The figure shows three views and two pictorial views of one solid part (mm, origin at its lowest corner). Answer the questions. A direction names the side the tool comes from. Coordinates: 2 decimals unless noted, no trailing zeros. Order: outer loops, then holes, each group sorted by start corner. A loop starts at its lowest first (then second) coordinate and runs counter-clockwise, first axis right, second up. Notation, with made-up numbers: (40, -36) -> (88, -36) arc R23 ccw to (88, -10) -> close; hole circle Ø10 at (-12.75, 8). An arc over 180 degrees is marked (long way). Return JSON: item names as keys, results as strings.
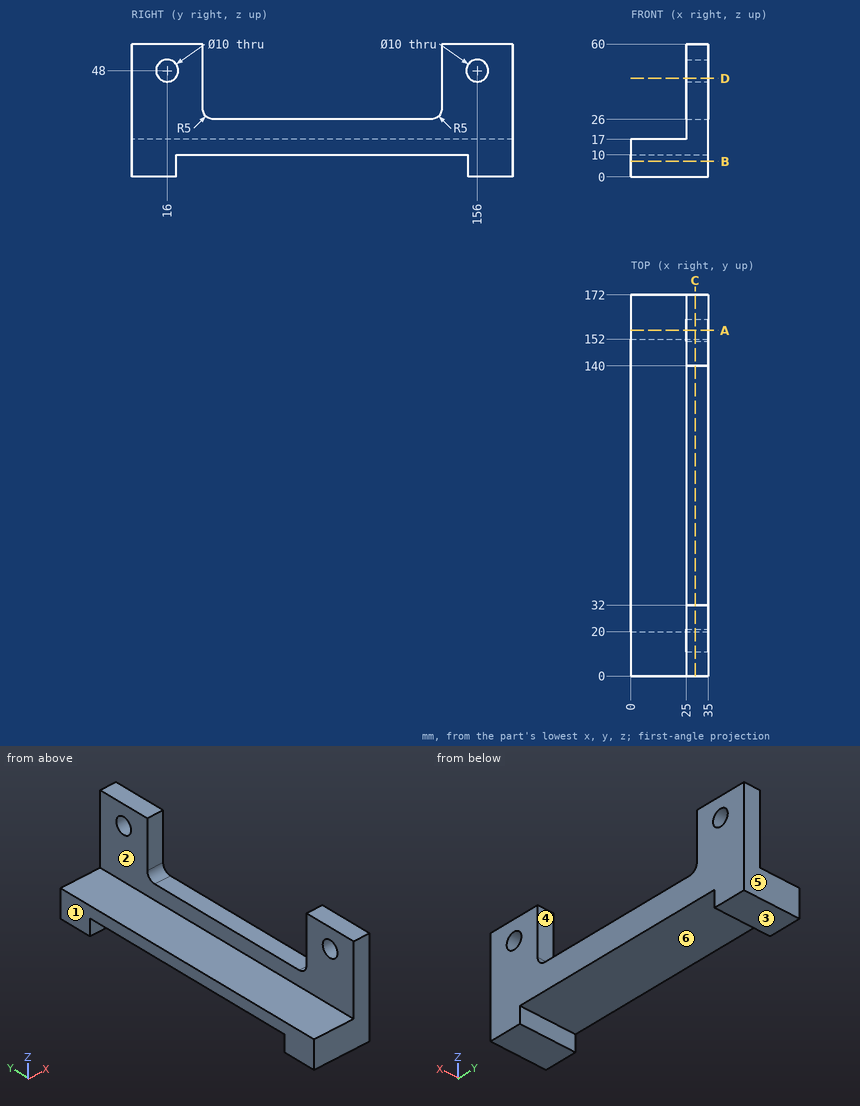
Item 1: Which of the six approach directions +Z, -Z, +X, -X, +Y, -Y give full straight-line access (tool end or side, diameter ignored) to the marked faces 1 and 2?
Answer list:
{"face 1": "+Z, -Z, -X, +Y, -Y", "face 2": "+Z, -X, +Y, -Y"}
Item 2: The part is cut by section C-C on x = 29. Determine the outline of the cut face in (y, z).
Answer list:
{"outline": "(0, 0) -> (20, 0) -> (20, 10) -> (152, 10) -> (152, 0) -> (172, 0) -> (172, 60) -> (140, 60) -> (140, 31) arc R5 cw to (135, 26) -> (37, 26) arc R5 cw to (32, 31) -> (32, 60) -> (0, 60) -> close; hole circle Ø10 at (16, 48); hole circle Ø10 at (156, 48)"}
Item 3: The part is cut by section B-B on z = 7. Determine the outline of the cut face in (x, y).
Answer list:
{"outline": "(0, 0) -> (35, 0) -> (35, 20) -> (0, 20) -> close; (0, 152) -> (35, 152) -> (35, 172) -> (0, 172) -> close"}
Item 4: The part is cut by section D-D on z = 44.5. Determine the outline of the cut face in (x, y).
Answer list:
{"outline": "(25, 0) -> (35, 0) -> (35, 12.43) -> (25, 12.43) -> close; (25, 19.57) -> (35, 19.57) -> (35, 32) -> (25, 32) -> close; (25, 140) -> (35, 140) -> (35, 152.43) -> (25, 152.43) -> close; (25, 159.57) -> (35, 159.57) -> (35, 172) -> (25, 172) -> close"}
Item 5: Find the intervals of material crossed by probe 1 along Z at (x, y) = (29, 156); probe 2 along Y at (x, z) = (27.5, 31); probe 3 along Z at (x, y) = (21, 54.5), in increasing order.
Answer list:
{"probe 1": "0 to 43, 53 to 60", "probe 2": "0 to 32, 140 to 172", "probe 3": "10 to 17"}
Item 6: Determine the mould class of the marked faces 3, 4, 5 and 6 for opening direction Y: pulls with the +Y half, pulls with the -Y half, needs draft (parallel to the pull), parting line crosses it, or undercut.
Answer list:
{"face 3": "needs draft", "face 4": "undercut", "face 5": "pulls with the +Y half", "face 6": "undercut"}
Item 7: The part is cut by section A-A on y = 156. Determine the outline of the cut face in (x, z), plus the area to 3 significant figures.
Answer list:
{"outline": "(0, 0) -> (35, 0) -> (35, 43) -> (25, 43) -> (25, 17) -> (0, 17) -> close; (25, 53) -> (35, 53) -> (35, 60) -> (25, 60) -> close", "area": "925 mm2"}
Item 8: Flat-ended cylindrical pins translate along their axes: pin 1 (12.5 mm diameter, centred on x = 16, y = 86.5, fed in from +Z); pin 2 (3 mm diameter, centred on x = 31, y = 72.5, fed in from +Z); pin 3 (6 mm diameter, centred on y = 156, z = 48, fed in from +X). Find the tip coordinate at first contact, or state that the pin passes through.
Answer list:
{"pin 1": "z = 17", "pin 2": "z = 26", "pin 3": "through"}
